```python
from build123d import *

# Parameters (mm, degrees)
SKETCH1_R           = 1.190625
BOSS_EXTRUDE4_DEPTH = 43.65625
BOSS_EXTRUDE5_DEPTH = 15.875
SKETCH7_W           = 4.699305321
SKETCH7_H           = 1.609279132
BOSS_EXTRUDE6_DEPTH = 18.161


with BuildPart() as part:
    # Sketch1 → Boss-Extrude4 (new body)
    with BuildSketch(Plane(origin=(0, 0, 0), x_dir=(1, 0, 0), z_dir=(0, 1, 0))):
        with BuildLine():
            ThreePointArc((1.961121792, 5.783909674), (1.616585512, 6.873597745), (1.500127735, 8.01050712))
            Line((1.500127735, 8.01050712), (1.500127735, 8.234009675))
            ThreePointArc((1.500127735, 8.234009675), (1.481529016, 8.278910955), (1.436627735, 8.297509675))
            Line((1.436627735, 8.297509675), (-2.865497265, 8.297509675))
            Line((-2.865497265, 8.297509675), (-3.262372265, 8.297509675))
            Line((-3.262372265, 8.297509675), (-3.262372265, 7.900634675))
            Line((-3.262372265, 7.900634675), (-3.262372265, -4.005615325))
            Line((-3.262372265, -4.005615325), (-3.262372265, -4.402490325))
            Line((-3.262372265, -4.402490325), (-2.865497265, -4.402490325))
            Line((-2.865497265, -4.402490325), (1.436627735, -4.402490325))
            ThreePointArc((1.436627735, -4.402490325), (1.481529016, -4.383891606), (1.500127735, -4.338990325))
            Line((1.500127735, -4.338990325), (1.500127735, -4.11548777))
            ThreePointArc((1.500127735, -4.11548777), (1.616585512, -2.978578396), (1.961121792, -1.888890325))
            ThreePointArc((1.961121792, -1.888890325), (2.755408878, 1.947509675), (1.961121792, 5.783909674))
        make_face()
        with Locations((-0.881122265, 1.947509675)):
            Circle(SKETCH1_R, mode=Mode.SUBTRACT)
    extrude(amount=BOSS_EXTRUDE4_DEPTH)

    # Sketch6 → Boss-Extrude5 (add)
    with BuildSketch(Plane.ZY.offset(3.262372265)):
        with BuildLine():
            Line((0.036865325, 3.175), (5.926490325, 3.175))
            ThreePointArc((5.926490325, 3.175), (5.971391606, 3.156401281), (5.989990325, 3.1115))
            Line((5.989990325, 3.1115), (5.989990325, 0.85725))
            ThreePointArc((5.989990325, 0.85725), (5.971391606, 0.812348719), (5.926490325, 0.79375))
            Line((5.926490325, 0.79375), (0.100365325, 0.79375))
            ThreePointArc((0.100365325, 0.79375), (0.055464045, 0.812348719), (0.036865325, 0.85725))
            Line((0.036865325, 0.85725), (0.036865325, 3.175))
        make_face()
    extrude(amount=BOSS_EXTRUDE5_DEPTH)

    # Sketch7 → Boss-Extrude6 (add)
    with BuildSketch(Plane.XZ):
        with Locations((-0.912719605, 5.207129891)):
            Rectangle(SKETCH7_W, SKETCH7_H)
    extrude(amount=-BOSS_EXTRUDE6_DEPTH)


solid = part.part
```
The listing builds one solid part. Answer for the finished solid, in the listing's coordinates (mm). A direction names the side the tool comes from. Coordinates: 2 decimals unless noted, no trailing zeros. Loops run counter-clockwise (first coordinate to the right, second up) from the corner with the lowest first, then second, coordinate; pieces in that order, holes last. Notation, with made-up numbers: (74.25, -39.5) -> (123.25, -39.5) arc R5 cw to (123.25, -33.5) -> close; hole circle Ø7 at (84.25, 81.5). An arc over 180 degrees is marked (long way). Use one line per item in the form item = value. Start each with the question number.
Item 1: Consider L1, parallel to Y at x = -10, z = 4.5 (3 decimals); L2, parallel to X at y = 22, z = -3; L3, parallel to X at y = 12.5, z = -2.5. Determine where each line is inside the solid, lowest interval first. Write a range as [from, to].
Item 2: A tool of negligible diameter and unlimited length cuts with its end or side. For faces 5 (the face through (1.437, 9, 5)), 6 (the face through (-11, 2, 0.037)), 7 (the face through (-1, 31, 4.402)), 8 (the face through (-11, 3.175, 3)), from which of +Z, -Z, +X, -X, +Y, -Y can it reach the whole face along a straight path? Write none if from no direction.
Item 3: The part is cut by section A-A on x = -2.5. Determine the outline of the cut face in (y, z), then the cut area to 3 significant figures.
Item 4: The part is cut by section D-D on z = 3. Determine the outline of the cut face in (x, y) (3 decimals).
Item 5: The part is cut by section B-B on z = -2.5. Determine the outline of the cut face in (x, y), then the cut area to 3 significant figures.
Item 6: The part is cut by section C-C on y = 32.5. Determine the outline of the cut face in (x, z).
Item 7: Flat-ended cylindrical pins translate along their axes: pin 1 Ø4.5 at (y, z) = (26, 0.5) entering from -X; pin 2 Ø1.5 at (y, z) = (34.5, 0) entering from +X; pin 3 Ø0.5 at (y, z) = (11, 5.5) entering from +X; pin 4 Ø4 at (x, y) = (-3.5, 14) entering from +Z. Find the tip coordinate at first contact, or state that the pin passes through.
Item 8: The mould has two halves that part along X. Classify faces 1 (the face through (1.62, 21.52, -6.86)), 2 (the face through (-1.139, 21.523, -0.785)), 3 (the face through (-19.137, 2, 3)), 4 (the face through (-1, 18.161, 5)): released by +X, released by -X, zero draft, split by the parting line, or undercut.
Answer key:
q1.L1 = [0.794, 3.175]
q1.L2 = [-3.26, -1.44], [-0.32, 2.7]
q1.L3 = [-3.26, -1.94], [0.17, 2.74]
q2.face_5 = +Z, +X, +Y, -Y
q2.face_6 = -Z, -X, +Y, -Y
q2.face_7 = +Z, +X, -X, +Y
q2.face_8 = +Z, -Z, -X, +Y
q3.outline = (0, -8.3) -> (43.66, -8.3) -> (43.66, 4.4) -> (18.16, 4.4) -> (18.16, 6.01) -> (0, 6.01) -> close
q3.area = 584 mm2
q4.outline = (-19.137, 0.794) -> (-3.262, 0.794) -> (-3.262, 0) -> (1.612, 0) -> (1.612, 43.656) -> (-3.262, 43.656) -> (-3.262, 3.175) -> (-19.137, 3.175) -> close
q5.outline = (-3.26, 0) -> (-1.94, 0) -> (-1.94, 43.66) -> (-3.26, 43.66) -> close; (0.17, 0) -> (2.74, 0) -> (2.74, 43.66) -> (0.17, 43.66) -> close
q5.area = 170 mm2
q6.outline = (-3.26, -8.3) -> (1.44, -8.3) arc R0.06 ccw to (1.5, -8.23) -> (1.5, -8.01) arc R5.61 cw to (1.96, -5.78) arc R9.66 ccw to (1.96, 1.89) arc R5.61 cw to (1.5, 4.12) -> (1.5, 4.34) arc R0.06 ccw to (1.44, 4.4) -> (-3.26, 4.4) -> close; hole circle Ø2.38 at (-0.88, -1.95)
q7.pin_1 = -3.26
q7.pin_2 = 2.68
q7.pin_3 = 1.44
q7.pin_4 = 6.01
q8.face_1 = released by +X
q8.face_2 = undercut
q8.face_3 = released by -X
q8.face_4 = zero draft
